from build123d import *

# Parameters (mm, degrees)
SKETCH1_W           = 15.2
SKETCH1_H           = 30.3
SKETCH1_W_2         = 13
SKETCH1_H_2         = 28.3
BOSS_EXTRUDE1_DEPTH = 13.1
SKETCH2_R           = 1
CUT_EXTRUDE1_DEPTH  = 26.143040787
SKETCH3_R           = 2.5
CUT_EXTRUDE2_DEPTH  = 34.874178957


with BuildPart() as part:
    # Sketch1 → Boss-Extrude1 (new body)
    with BuildSketch(Plane(origin=(0, 0, 0), x_dir=(1, 0, 0), z_dir=(0, 1, 0))):
        Rectangle(SKETCH1_W, SKETCH1_H)
        Rectangle(SKETCH1_W_2, SKETCH1_H_2, mode=Mode.SUBTRACT)
    extrude(amount=BOSS_EXTRUDE1_DEPTH)

    # Sketch2 → Cut-Extrude1 (cut, through all)
    with BuildSketch(Plane(origin=(7.6, 0, 0), x_dir=(0, 0, -1), z_dir=(1, 0, 0))):
        with Locations((-7.5, 6.55)):
            Circle(SKETCH2_R)
        with Locations((7.5, 6.55)):
            Circle(SKETCH2_R)
    extrude(amount=-CUT_EXTRUDE1_DEPTH, mode=Mode.SUBTRACT)

    # Sketch3 → Cut-Extrude2 (cut, through all)
    with BuildSketch(Plane.XY.offset(15.15)):
        with Locations((0, 6.55)):
            Circle(SKETCH3_R)
    extrude(amount=-CUT_EXTRUDE2_DEPTH, mode=Mode.SUBTRACT)


solid = part.part
The model under review builds one solid part; all positions refer to its coordinate system, in mm. A direction names the side the tool comes from. Round coordinates to 2 decimals unless told otherwise and drop trailing zeros. Loops run counter-clockwise (first coordinate to the right, second up) from the corner with the lowest first, then second, coordinate; pieces in that order, holes last. Notation, with made-up numbers: M -39.75,19.25 L -18.75,19.25 A22 cw -18.75,52.25 Z; hole C -33.5,64.25 d11. An arc over 180 degrees is marked long. Answer as CSV lines item,"result".
1. For faces 1 (the face through (-7, 13.1, -1)), 2 (the face through (-6.5, 6, 0)), list the 3-axis set-ups (+Z, -Z, +X, -X, +Y, -Y) from which the entire face can be reached by the end or side of a thin tool; tool diameter is ignored.
Outcome:
face 1,"+Z, -Z, +X, -X, +Y"
face 2,"+Y, -Y"
2. We need section B-B (x = 0). Give the boundary of the cut face in (y, z).
Outcome:
outline,"M 0,-15.15 L 4.05,-15.15 L 4.05,-14.15 L 0,-14.15 Z; M 0,14.15 L 4.05,14.15 L 4.05,15.15 L 0,15.15 Z; M 9.05,-15.15 L 13.1,-15.15 L 13.1,-14.15 L 9.05,-14.15 Z; M 9.05,14.15 L 13.1,14.15 L 13.1,15.15 L 9.05,15.15 Z"
3. We need section C-C (z = 7.5). Give the boundary of the cut face in (x, y), plus the area to 3 significant figures.
Outcome:
outline,"M -7.6,0 L -6.5,0 L -6.5,5.55 L -7.6,5.55 Z; M -7.6,7.55 L -6.5,7.55 L -6.5,13.1 L -7.6,13.1 Z; M 6.5,0 L 7.6,0 L 7.6,5.55 L 6.5,5.55 Z; M 6.5,7.55 L 7.6,7.55 L 7.6,13.1 L 6.5,13.1 Z"
area,"24.4 mm2"
4. We need section D-D (y = 6.55). Count the separate pieces of the cut face and the enclosed holes in it, plus the area to 3 significant figures.
Outcome:
separate pieces,"6"
enclosed holes,"0"
area,"73.9 mm2"
5. To check wall thickness, follow L1, parallel to Y at x = -7.05, z = -7.5; L2, parallel to X at y = 9, z = -8; L3, parallel to Z at x = 5.5, y = 5. State the ranges of each line that lie inside material, in increasing order. Write a range as [from, to].
Outcome:
L1,"y = [0, 5.55], [7.55, 13.1]"
L2,"x = [-7.6, -6.5], [6.5, 7.6]"
L3,"z = [-15.15, -14.15], [14.15, 15.15]"
6. We need section A-A (z = -6). Give the boundary of the cut face in (x, y).
Outcome:
outline,"M -7.6,0 L -6.5,0 L -6.5,13.1 L -7.6,13.1 Z; M 6.5,0 L 7.6,0 L 7.6,13.1 L 6.5,13.1 Z"
7. Draft analysis for pull direction X (two halves, no side actions). For faces 3 (the face through (-7.04, 7.54, -7.37)), 4 (the face through (-7.6, 6, 0)), 5 (the face through (-3, 6, -14.15)), 6 (the face through (7.6, 6, 0)), state which applies: pulls with the +X half, pulls with the -X half, needs draft (parallel to the pull), parting line crosses it, or undercut.
Outcome:
face 3,"needs draft"
face 4,"pulls with the -X half"
face 5,"undercut"
face 6,"pulls with the +X half"
